```python
from build123d import *

# Parameters (mm, degrees)
SKETCH1_W           = 42.5
SKETCH1_H           = 40
BOSS_EXTRUDE1_DEPTH = 2
SKETCH2_R           = 1.5
CUT_EXTRUDE1_DEPTH  = 4
SKETCH3_R           = 11
CUT_EXTRUDE2_DEPTH  = 4
SKETCH4_W           = 42.5
SKETCH4_H           = 4
BOSS_EXTRUDE2_DEPTH = 15
SKETCH7_R           = 1.5
CUT_EXTRUDE3_DEPTH  = 10


with BuildPart() as part:
    # Sketch1 → Boss-Extrude1 (new, symmetric)
    with BuildSketch(Plane.XY):
        Rectangle(SKETCH1_W, SKETCH1_H)
    extrude(amount=BOSS_EXTRUDE1_DEPTH, both=True)

    # Sketch2 → Cut-Extrude1 (cut)
    with BuildSketch(Plane(origin=(0, 0, -2), x_dir=(-1, 0, 0), z_dir=(0, 0, -1))):
        with Locations((-16.75, 15.5)):
            Circle(SKETCH2_R)
        with Locations((14.25, 15.5)):
            Circle(SKETCH2_R)
        with Locations((14.25, -15.5)):
            Circle(SKETCH2_R)
        with Locations((-16.75, -15.5)):
            Circle(SKETCH2_R)
    extrude(amount=-CUT_EXTRUDE1_DEPTH, mode=Mode.SUBTRACT)

    # Sketch3 → Cut-Extrude2 (cut)
    with BuildSketch(Plane.XY.offset(2)):
        with Locations((1.25, 0)):
            Circle(SKETCH3_R)
    extrude(amount=-CUT_EXTRUDE2_DEPTH, mode=Mode.SUBTRACT)

    # Sketch4 → Boss-Extrude2 (add)
    with BuildSketch(Plane(origin=(0, 20, 0), x_dir=(1, 0, 0), z_dir=(0, 1, 0))):
        Rectangle(SKETCH4_W, SKETCH4_H)
    extrude(amount=BOSS_EXTRUDE2_DEPTH)

    # Sketch7 → Cut-Extrude3 (cut)
    with BuildSketch(Plane.XY.offset(2)):
        with Locations((-7.894013049, 23.945501151)):
            Circle(SKETCH7_R)
        with Locations((10.105662158, 24.053632735)):
            Circle(SKETCH7_R)
        with Locations((10.303903396, -8.945771811)):
            Circle(SKETCH7_R)
        with Locations((-7.695771811, -9.053903396)):
            Circle(SKETCH7_R)
    extrude(amount=-CUT_EXTRUDE3_DEPTH, mode=Mode.SUBTRACT)


solid = part.part
```
Geometry check sheet. Reference: the model listing, model coordinates, mm. Coordinates: 2 decimals unless noted, no trailing zeros. Order: outer loops, then holes, each group sorted by start corner. A loop starts at its lowest first (then second) coordinate and runs counter-clockwise, first axis right, second up. Notation, with made-up numbers: (-4, -32) - (41, -32) arc R16 ccw to (41, -19) - close; hole circle Ø11 at (12, -26). An arc over 180 degrees is marked (long way). Use one line per item in the form item = value.
1. Section check C-C (x = 16.75). Record the boundary of the cut face in (y, z).
Here are the results:
outline = (-20, -2) - (-17, -2) - (-17, 2) - (-20, 2) - close; (-14, -2) - (14, -2) - (14, 2) - (-14, 2) - close; (17, -2) - (35, -2) - (35, 2) - (17, 2) - close
2. Section check B-B (y = 15.5). Record the boundary of the cut face in (x, z).
Here are the results:
outline = (-21.25, -2) - (-15.75, -2) - (-15.75, 2) - (-21.25, 2) - close; (-12.75, -2) - (15.25, -2) - (15.25, 2) - (-12.75, 2) - close; (18.25, -2) - (21.25, -2) - (21.25, 2) - (18.25, 2) - close
3. Section check D-D (y = 0). Record the boundary of the cut face in (x, z).
Here are the results:
outline = (-21.25, -2) - (-9.75, -2) - (-9.75, 2) - (-21.25, 2) - close; (12.25, -2) - (21.25, -2) - (21.25, 2) - (12.25, 2) - close
4. Section check A-A (x = 1.25). Record the boundary of the cut face in (y, z).
Here are the results:
outline = (-20, -2) - (-11, -2) - (-11, 2) - (-20, 2) - close; (11, -2) - (35, -2) - (35, 2) - (11, 2) - close
5. Draft check along Y on faces 1 (the face through (-21.25, 7, 0)), 2 (the face through (0, 35, 0)), 3 (the face through (-8.089, 25.433, 0.028)), 4 (the face through (-12.75, 15.57, -0.03)). Enter one of: pulls with the +Y half, pulls with the -Y half, needs draft (parallel to the pull), parting line crosses it, or undercut.
Here are the results:
face_1 = needs draft
face_2 = pulls with the +Y half
face_3 = undercut
face_4 = undercut
6. Scan lines: line 1 (Y direction, x = 16.75, z = -0.7); line 2 (Y direction, x = 9.5, z = 0.1); line 3 (Y direction, x = 18, z = -1.8). Record each from-to range of solid material in increasing order.
Here are the results:
line_1 = -20 to -17, -14 to 14, 17 to 35
line_2 = -20 to -10.21, -7.68 to -7.28, 7.28 to 22.68, 25.43 to 35
line_3 = -20 to -16.33, -14.67 to 14.67, 16.33 to 35
